Check sheet for the modelled part. Datum: model origin and axes. Units: mm. A direction names the side the tool comes from. Give positions to 0.01 mm unless a question says otherwise; leave off trailing zeros. Write each loop counter-clockwise with the first axis right and the second up, starting at its lowest first coordinate (ties: lowest second). Pieces come first, ordered by that corner, then holes. Notation, with made-up numbers: (54, 58.25) - (60, 58.25) arc R30 ccw to (60, 86.25) - close; hole circle Ø2 at (-13, -1). An arc over 180 degrees is marked (long way). Return JSON: item names as keys, results as strings. Group by question number.
```python
from build123d import *

# Parameters (mm, degrees)
F0_R     = 25
F0_R_2   = 21
F1_DEPTH = 32
F2_ANGLE = 165
F4_DEPTH = 250


with BuildPart() as f1:
    # F0 (on Front) → F1 (new body, symmetric)
    with BuildSketch(Plane.XZ):
        Circle(F0_R)
        Circle(F0_R_2, mode=Mode.SUBTRACT)
    extrude(amount=F1_DEPTH, both=True)


with BuildPart() as f1_1:
    # F2: moved
    add(f1.part.rotate(Axis((0, 0, -29.1226431727), (0, 0, -1)), F2_ANGLE))

    # F3 (on Right) → F4 (join)
    with BuildSketch(Plane.YZ):
        with BuildLine():
            ThreePointArc((-26.0919821262, -14), (-24.3346228134, -18.2426406871), (-20.0919821262, -20))
            Line((-20.0919821262, -20), (7.9080178738, -20))
            ThreePointArc((7.9080178738, -20), (12.1506585609, -18.2426406871), (13.9080178738, -14))
            Line((13.9080178738, -14), (13.9080178738, 14))
            ThreePointArc((13.9080178738, 14), (12.1506585609, 18.2426406871), (7.9080178738, 20))
            Line((7.9080178738, 20), (-20.0919821262, 20))
            ThreePointArc((-20.0919821262, 20), (-24.3346228134, 18.2426406871), (-26.0919821262, 14))
            Line((-26.0919821262, 14), (-26.0919821262, -14))
        make_face()
        with BuildLine():
            Line((7.9080178738, -17), (-20.0919821262, -17))
            ThreePointArc((-20.0919821262, -17), (-22.2133024698, -16.1213203436), (-23.0919821262, -14))
            Line((-23.0919821262, -14), (-23.0919821262, 14))
            ThreePointArc((-23.0919821262, 14), (-22.2133024698, 16.1213203436), (-20.0919821262, 17))
            Line((-20.0919821262, 17), (7.9080178738, 17))
            ThreePointArc((7.9080178738, 17), (10.0293382173, 16.1213203436), (10.9080178738, 14))
            Line((10.9080178738, 14), (10.9080178738, -14))
            ThreePointArc((10.9080178738, -14), (10.0293382173, -16.1213203436), (7.9080178738, -17))
        make_face(mode=Mode.SUBTRACT)
    extrude(amount=-F4_DEPTH)


solid = f1_1.part
```
Item 1: Material ranges on line 1 along Z through (x, y) = (-155, -14); line 2 along Y through (x, z) = (-67, -2.5); line 3 along X through (y, z) = (-22.5, 3), recorded low to high. Write a range as from..to.
Item 2: Section check B-B on z = -2.5. Record the cut outline in (x, y).
Item 3: Depth check by flat-ended pin: pin 1 (10 mm diameter, centred on x = -176, z = -6, fed in from -Y); pin 2 (16.5 mm diameter, centred on x = -6, y = -7, fed in from -Z); pin 3 (10 mm diameter, centred on x = -13, y = 8, fed in from -Z). Enter the tip coordinate at first touch or a pass-through.
Item 4: Section check A-A on x = -65.5. Record the cut outline in (y, z), plus the area to 3 significant figures.
Item 5: Mould release check, pull along Z, two halves, no side actions. Record for faces 1 (the face through (-131, -26.092, 0)), 2 (the face through (-132.2, 12.1, -18.29)), 3 (the face through (-128, -6, 20)), 4 (the face through (-3.518, -25.557, -16.476)): +Z half, -Z half, draft (parallel to the pull), parting line (faces both ways), or undercut.
Item 6: Access from +Z, -Z, +X, -X, +Y, -Y to the whole of each face (thin tool, end or side, straight path). Record for faces 5 (the face through (-2.8, 32.38, 20.49)), 6 (the face through (-130, -6, 17)), 7 (the face through (-3, -3, 20)), 8 (the face through (-128.309, -24.288, 18.289)).
Reply:
{
 "1": {"line 1": "-20..-17, 17..20", "line 2": "-26.09..-23.09, 10.91..13.91", "line 3": "-19.67..-15.49, 27.55..31.72"},
 "2": {"outline": "(-250, -26.09) - (-18.76, -26.09) - (-15.74, -37.35) - (-11.86, -36.31) - (-14.59, -26.09) - (0, -26.09) - (0, -23.09) - (-15.4, -23.09) - (-24.51, 10.91) - (0, 10.91) - (0, 13.91) - (-25.31, 13.91) - (-28.42, 25.51) - (-32.31, 24.47) - (-29.48, 13.91) - (-250, 13.91) - (-250, 10.91) - (-28.67, 10.91) - (-19.56, -23.09) - (-250, -23.09) - close; (11.86, 36.31) - (28.42, -25.51) - (32.31, -24.47) - (15.74, 37.35) - close"},
 "3": {"pin 1": "y = -26.09", "pin 2": "z = -25", "pin 3": "z = -24.39"},
 "4": {"outline": "(-26.09, -14) arc R6 ccw to (-20.09, -20) - (7.91, -20) arc R6 ccw to (13.91, -14) - (13.91, 14) arc R6 ccw to (7.91, 20) - (-20.09, 20) arc R6 ccw to (-26.09, 14) - close; hole (-23.09, -14) arc R3 ccw to (-20.09, -17) - (7.91, -17) arc R3 ccw to (10.91, -14) - (10.91, 14) arc R3 ccw to (7.91, 17) - (-20.09, 17) arc R3 ccw to (-23.09, 14) - close", "area": "421 mm²"},
 "5": {"face 1": "draft", "face 2": "-Z half", "face 3": "+Z half", "face 4": "undercut"},
 "6": {"face 5": "+Z, -Z, -X, +Y", "face 6": "-X", "face 7": "none", "face 8": "+Z, -X, -Y"}
}
